```python
from build123d import *

# Parameters (mm, degrees)
SKETCH_1_W                  = 143.42529591
SKETCH_1_H                  = 80.35
SKETCH_1_R                  = 1.5
SKETCH_1_W_2                = 127.420983087
SKETCH_1_H_2                = 74.55
EXTRUDE_1_DEPTH             = 3
SKETCH_2_W                  = 131.42529591
SKETCH_2_H                  = 5
SKETCH_2_R                  = 1.5
EXTRUDE_2_DEPTH             = 2.8
SKETCH_3_R                  = 1.5
CUT_EXTRUDE_1_DEPTH         = 10
SKETCH_4_W                  = 6
SKETCH_4_H                  = 8
EXTRUDE_3_DEPTH             = 10
SKETCH_5_W                  = 54.485918212
SKETCH_5_H                  = 8
EXTRUDE_4_DEPTH             = 3
FILLET_1_R                  = 10
FILLET_2_R                  = 10
SKETCH_6_R                  = 1.5
CUT_EXTRUDE_2_DEPTH         = 3
EXTRUDE_5_DEPTH             = 2.8
SKETCH_8_W                  = 42.5
SKETCH_8_H                  = 8
SKETCH_8_H_2                = 10.9
SKETCH_8_R                  = 1.5
CUT_EXTRUDE_3_DEPTH         = 3
EXTRUDE_6_REACH             = 127.55
EXTRUDE_6_DIRECTION_2_DEPTH = 2.8
SKETCH_11_R                 = 1.5
SKETCH_11_R_2               = 1.490339558
CUT_EXTRUDE_4_DEPTH         = 3
EXTRUDE_START               = -3
EXTRUDE_7_DEPTH             = 3


with BuildPart() as part:
    # 草图1 → 凸台-拉伸1 (new body)
    with BuildSketch(Plane.XY):
        with Locations((-13.602517363, 6.11984421)):
            Rectangle(SKETCH_1_W, SKETCH_1_H)
        with Locations((55.610130592, -24.05515579)):
            Circle(SKETCH_1_R, mode=Mode.SUBTRACT)
        with Locations((55.610130592, 6.11984421)):
            Circle(SKETCH_1_R, mode=Mode.SUBTRACT)
        with Locations((55.610130592, 36.29484421)):
            Circle(SKETCH_1_R, mode=Mode.SUBTRACT)
        with Locations((-82.810852495, -24.05515579)):
            Circle(SKETCH_1_R, mode=Mode.SUBTRACT)
        with Locations((-82.810852495, 6.11984421)):
            Circle(SKETCH_1_R, mode=Mode.SUBTRACT)
        with Locations((-82.810852495, 36.29484421)):
            Circle(SKETCH_1_R, mode=Mode.SUBTRACT)
        with Locations((-13.600360952, 6.21984421)):
            Rectangle(SKETCH_1_W_2, SKETCH_1_H_2, mode=Mode.SUBTRACT)
    extrude(amount=EXTRUDE_1_DEPTH)

    # 草图2 → 凸台-拉伸2 (add)
    with BuildSketch(Plane(origin=(0, 46.29484421, 0), x_dir=(1, 0, 0), z_dir=(0, 1, 0))):
        with Locations((-13.602517363, -5.5)):
            Rectangle(SKETCH_2_W, SKETCH_2_H)
        with Locations(Location((-21.702517363, -5, 0), (0, 0, 180))):
            Circle(SKETCH_2_R, mode=Mode.SUBTRACT)
    extrude(amount=-EXTRUDE_2_DEPTH)

    # 草图3 → 切除-拉伸1 (cut)
    with BuildSketch(Plane(origin=(0, 46.29484421, 0), x_dir=(1, 0, 0), z_dir=(0, 1, 0))):
        with Locations(Location((0.240439338, -5, 0), (0, 0, 270))):
            Circle(SKETCH_3_R)
        with Locations(Location((-43.645478874, -5, 0), (0, 0, 270))):
            Circle(SKETCH_3_R)
    extrude(amount=-CUT_EXTRUDE_1_DEPTH, mode=Mode.SUBTRACT)

    # 草图4 → 凸台-拉伸3 (add)
    with BuildSketch(Plane(origin=(0, 46.29484421, 0), x_dir=(1, 0, 0), z_dir=(0, 1, 0))):
        with Locations((8.540439338, -4)):
            Rectangle(SKETCH_4_W, SKETCH_4_H)
        with Locations((-51.945478874, -4)):
            Rectangle(SKETCH_4_W, SKETCH_4_H)
    extrude(amount=EXTRUDE_3_DEPTH)

    # 草图5 → 凸台-拉伸4 (add)
    with BuildSketch(Plane(origin=(0, 56.29484421, 0), x_dir=(1, 0, 0), z_dir=(0, 1, 0))):
        with Locations((-21.702519768, -4)):
            Rectangle(SKETCH_5_W, SKETCH_5_H)
    extrude(amount=-EXTRUDE_4_DEPTH)

    # 圆角1
    fillet_1_edges = [part.edges().sort_by_distance(p)[0] for p in [
        (11.540439338, 46.29484421, 4),
        (-54.945478874, 46.29484421, 4),
    ]]
    fillet(fillet_1_edges, radius=FILLET_1_R - 0.0001)  # a hair under: the kernel refuses the full size

    # 圆角2
    fillet_2_edges = [part.edges().sort_by_distance(p)[0] for p in [
        (-54.945478874, 56.29484421, 4),
        (11.540439338, 56.29484421, 4),
    ]]
    fillet(fillet_2_edges, radius=FILLET_2_R)

    # 草图6 → 切除-拉伸2 (cut)
    with BuildSketch(Plane(origin=(0, 56.29484421, 0), x_dir=(1, 0, 0), z_dir=(0, 1, 0))):
        with Locations(Location((0.240439338, -5, 0), (0, 0, 270))):
            Circle(SKETCH_6_R)
        with Locations(Location((-21.702517363, -5, 0), (0, 0, 180))):
            Circle(SKETCH_6_R)
        with Locations(Location((-43.645478874, -5, 0), (0, 0, 270))):
            Circle(SKETCH_6_R)
    extrude(amount=-CUT_EXTRUDE_2_DEPTH, mode=Mode.SUBTRACT)

    # 草图7 → 凸台-拉伸5 (add)
    with BuildSketch(Plane(origin=(0, 46.29484421, 0), x_dir=(1, 0, 0), z_dir=(0, 1, 0))):
        with BuildLine():
            Line((52.110130592, -3), (-79.315165318, -3))
            ThreePointArc((-79.315165318, -3), (-71.408587337, -30.249323597), (-49.947485102, -48.808976146))
            ThreePointArc((-49.947485102, -48.808976146), (-47.931875984, -49.474706171), (-45.821160639, -49.7))
            Line((-45.821160639, -49.7), (3.801028521, -49.7))
            ThreePointArc((3.801028521, -49.7), (4.482979053, -49.676720076), (5.161754433, -49.606988694))
            ThreePointArc((5.161754433, -49.606988694), (36.42646247, -34.151078405), (52.110130592, -3))
        make_face()
    extrude(amount=-EXTRUDE_5_DEPTH)

    # 草图8 → 切除-拉伸3 (cut)
    with BuildSketch(Plane(origin=(0, 46.29484421, 0), x_dir=(1, 0, 0), z_dir=(0, 1, 0))):
        with BuildLine():
            Line((52.110130592, -8), (52.110130592, -3))
            ThreePointArc((52.110130592, -3), (51.686965751, -5.511139637), (51.148017839, -8))
            Line((51.148017839, -8), (52.110130592, -8))
        make_face()
        with BuildLine():
            ThreePointArc((-79.091069545, -8), (-79.253197971, -5.766605102), (-79.315165318, -3.528190833))
            Line((-79.315165318, -3.528190833), (-79.315165318, -8))
            Line((-79.315165318, -8), (-79.091069545, -8))
        make_face()
        with BuildLine():
            Line((-79.315165318, -3.528190833), (-79.315165318, -3))
            ThreePointArc((-79.315165318, -3), (-79.315862787, -3.264095416), (-79.315165318, -3.528190833))
        make_face()
        with Locations((-21.687503936, -23.091321672)):
            Rectangle(SKETCH_8_W, SKETCH_8_H)
        with Locations((-21.687503936, -13.641321672)):
            Rectangle(SKETCH_8_W, SKETCH_8_H_2)
        with Locations(Location((0.240439338, -5, 0), (0, 0, 270))):
            Circle(SKETCH_8_R)
        with Locations(Location((-43.645478874, -5, 0), (0, 0, 270))):
            Circle(SKETCH_8_R)
        with Locations(Location((-21.702517363, -5, 0), (0, 0, 270))):
            Circle(SKETCH_8_R)
    extrude(amount=-CUT_EXTRUDE_3_DEPTH, mode=Mode.SUBTRACT)

    # 凸台-拉伸6: up to this face of the body (flat: up to its plane)
    extrude_6_end = Plane(part.part.faces().sort_by_distance((-13.602517363, -34.05515579, 1.5))[0])
    # 草图9 → 凸台-拉伸6 (add, up to the picked face)
    with BuildSketch(Plane.XZ.offset(-43.49484421), mode=Mode.PRIVATE) as extrude_6_sk1:
        with BuildLine():
            ThreePointArc((-45.821160639, 49.7), (-47.931875984, 49.474706171), (-49.947485102, 48.808976146))
            ThreePointArc((-49.947485102, 48.808976146), (-71.265466668, 30.471277082), (-79.315165318, 3.528190833))
            Line((-79.315165318, 3.528190833), (-79.315165318, 3))
            Line((-79.315165318, 3), (-77.284463301, 3))
            Line((-77.284463301, 3), (-77.284463301, 5))
            ThreePointArc((-77.284463301, 5), (-69.179280492, 30.001857642), (-49.122220209, 46.987180917))
            ThreePointArc((-49.122220209, 46.987180917), (-47.509732915, 47.519764937), (-45.821160639, 47.7))
            Line((-45.821160639, 47.7), (3.801028521, 47.7))
            ThreePointArc((3.801028521, 47.7), (4.346588947, 47.681376061), (4.889609251, 47.625590956))
            ThreePointArc((4.889609251, 47.625590956), (34.185844829, 33.539377025), (49.748453895, 5))
            Line((49.748453895, 5), (50.110130592, 3))
            Line((50.110130592, 3), (52.615296987, 3))
            ThreePointArc((52.615296987, 3), (38.28835989, 32.947499211), (9.430945753, 49.359795972))
            ThreePointArc((9.430945753, 49.359795972), (7.851760578, 49.614706494), (6.254409581, 49.7))
            Line((6.254409581, 49.7), (-45.821160639, 49.7))
        make_face()
    extrude_6_tool1 = split(extrude(extrude_6_sk1.sketch, amount=EXTRUDE_6_REACH, mode=Mode.PRIVATE), bisect_by=extrude_6_end, keep=Keep.BOTH, mode=Mode.PRIVATE)
    add(extrude_6_tool1.solids().sort_by(Axis((-47.636477, 43.494844, 48.106717), (0, -1, 0)))[0])

    # 草图9 → 凸台-拉伸6 direction 2 (add)
    with BuildSketch(Plane.XZ.offset(-43.49484421)):
        with BuildLine():
            ThreePointArc((-45.821160639, 49.7), (-47.931875984, 49.474706171), (-49.947485102, 48.808976146))
            ThreePointArc((-49.947485102, 48.808976146), (-71.265466668, 30.471277082), (-79.315165318, 3.528190833))
            Line((-79.315165318, 3.528190833), (-79.315165318, 3))
            Line((-79.315165318, 3), (-77.284463301, 3))
            Line((-77.284463301, 3), (-77.284463301, 5))
            ThreePointArc((-77.284463301, 5), (-69.179280492, 30.001857642), (-49.122220209, 46.987180917))
            ThreePointArc((-49.122220209, 46.987180917), (-47.509732915, 47.519764937), (-45.821160639, 47.7))
            Line((-45.821160639, 47.7), (3.801028521, 47.7))
            ThreePointArc((3.801028521, 47.7), (4.346588947, 47.681376061), (4.889609251, 47.625590956))
            ThreePointArc((4.889609251, 47.625590956), (34.185844829, 33.539377025), (49.748453895, 5))
            Line((49.748453895, 5), (50.110130592, 3))
            Line((50.110130592, 3), (52.615296987, 3))
            ThreePointArc((52.615296987, 3), (38.28835989, 32.947499211), (9.430945753, 49.359795972))
            ThreePointArc((9.430945753, 49.359795972), (7.851760578, 49.614706494), (6.254409581, 49.7))
            Line((6.254409581, 49.7), (-45.821160639, 49.7))
        make_face()
    extrude(amount=-EXTRUDE_6_DIRECTION_2_DEPTH)

    # 草图11 → 切除-拉伸4 (cut)
    with BuildSketch(Plane(origin=(0, 0, 47.7), x_dir=(-1, 0, 0), z_dir=(0, 0, -1))):
        with Locations((15.702514958, 40.59484421)):
            Circle(SKETCH_11_R)
        with Locations((27.702514958, 40.59484421)):
            Circle(SKETCH_11_R)
        with Locations((15.702514958, 28.59484421)):
            Circle(SKETCH_11_R)
        with Locations((27.702514958, 28.59484421)):
            Circle(SKETCH_11_R_2)
        with Locations((27.702514958, 16.59484421)):
            Circle(SKETCH_11_R)
        with Locations((15.702514958, 16.59484421)):
            Circle(SKETCH_11_R)
    extrude(amount=-CUT_EXTRUDE_4_DEPTH, mode=Mode.SUBTRACT)

    # 草图12 → 凸台-拉伸7 (add)
    with BuildSketch(Plane.XZ.offset(34.05515579).offset(EXTRUDE_START)):
        with BuildLine():
            Line((50.110130592, 3), (-77.284463301, 3))
            Line((-77.284463301, 3), (-77.284463301, 5))
            ThreePointArc((-77.284463301, 5), (-69.179280492, 30.001857642), (-49.122220209, 46.987180917))
            ThreePointArc((-49.122220209, 46.987180917), (-47.509732915, 47.519764937), (-45.821160639, 47.7))
            Line((-45.821160639, 47.7), (3.801028521, 47.7))
            ThreePointArc((3.801028521, 47.7), (4.346588947, 47.681376061), (4.889609251, 47.625590956))
            ThreePointArc((4.889609251, 47.625590956), (34.185844829, 33.539377025), (49.748453895, 5))
            Line((49.748453895, 5), (50.110130592, 3))
        make_face()
        with BuildLine():
            Line((50.110130592, 3), (52.110130592, 3))
            Line((52.110130592, 3), (52.615296987, 3))
            ThreePointArc((52.615296987, 3), (38.28835989, 32.947499211), (9.430945753, 49.359795972))
            ThreePointArc((9.430945753, 49.359795972), (7.851760578, 49.614706494), (6.254409581, 49.7))
            Line((6.254409581, 49.7), (3.801028521, 49.7))
            Line((3.801028521, 49.7), (-45.821160639, 49.7))
            ThreePointArc((-45.821160639, 49.7), (-47.931875984, 49.474706171), (-49.947485102, 48.808976146))
            ThreePointArc((-49.947485102, 48.808976146), (-71.265466668, 30.471277082), (-79.315165318, 3.528190833))
            Line((-79.315165318, 3.528190833), (-79.315165318, 3))
            Line((-79.315165318, 3), (-77.284463301, 3))
            Line((-77.284463301, 3), (-77.284463301, 5))
            ThreePointArc((-77.284463301, 5), (-69.179280492, 30.001857642), (-49.122220209, 46.987180917))
            ThreePointArc((-49.122220209, 46.987180917), (-47.509732915, 47.519764937), (-45.821160639, 47.7))
            Line((-45.821160639, 47.7), (3.801028521, 47.7))
            ThreePointArc((3.801028521, 47.7), (4.346588947, 47.681376061), (4.889609251, 47.625590956))
            ThreePointArc((4.889609251, 47.625590956), (34.185844829, 33.539377025), (49.748453895, 5))
            Line((49.748453895, 5), (50.110130592, 3))
        make_face()
    extrude(amount=EXTRUDE_7_DEPTH)


solid = part.part
```
Verification items for the finished model (mm, model axes). A direction names the side the tool comes from. Coordinates: 2 decimals unless noted, no trailing zeros. Loops run counter-clockwise (first coordinate to the right, second up) from the corner with the lowest first, then second, coordinate; pieces in that order, holes last. Notation, with made-up numbers: (11, 54.5) -> (40, 54.5) arc R24 ccw to (40, 90.5) -> close; hole circle Ø10 at (12.25, 29). An arc over 180 degrees is marked (long way). Answer in a Markdown table with one row per item.
1) Section check A-A (x = -34.5). Record the cut outline in (y, z).
The answers:
| item | result |
|---|---|
| outline | (-34.06, 0) -> (-31.06, 0) -> (-31.06, 47.7) -> (43.49, 47.7) -> (43.49, 27.09) -> (46.29, 27.09) -> (46.29, 49.7) -> (-34.06, 49.7) -> close; (43.49, 0) -> (46.29, 0) -> (46.29, 8.19) -> (43.49, 8.19) -> close; (53.29, 0) -> (56.29, 0) -> (56.29, 8) -> (53.29, 8) -> close |
2) Draft check along Z on faces 5 (the face through (-22, 45, 27.091)), 6 (the face through (-15, 46.295, 30)), 7 (the face through (-19, 7, 49.7)). Enter one of: released by +Z, released by -Z, zero draft, split by the parting line, or undercut.
The answers:
| item | result |
|---|---|
| face 5 | undercut |
| face 6 | zero draft |
| face 7 | released by +Z |
3) Depth check by flat-ended pin: P1, Ø3, axis at y = 45.5, z = 16.5, coming from the -X side; P2, Ø12, axis at x = -67, z = 6.5, coming from the +Y side; P3, Ø14.5, axis at x = 13, z = 31, coming from the +Y side; P4, Ø5, axis at x = 55.61, y = 36.29, coming from the -Z side. Enter the tip coordinate at first touch or a pass-through.
The answers:
| item | result |
|---|---|
| P1 | stops at x = -77.92 |
| P2 | stops at y = 47.11 |
| P3 | stops at y = 46.29 |
| P4 | stops at z = 0 |
4) Access from +Z, -Z, +X, -X, +Y, -Y to the whole of each face (thin tool, end or side, straight path). Record for faces 1 (the face through (-22, 45, 8.191)), 2 (the face through (5.54, 50, 4)), 3 (the face through (-21, 7, 47.7)), 4 (the face through (-22, 54, 8)).
The answers:
| item | result |
|---|---|
| face 1 | +Y |
| face 2 | +Z, -Z |
| face 3 | -Z |
| face 4 | +Z, +X, -X, +Y |
5) Section check B-B (z = 32). Record the cut outline in (x, y).
The answers:
| item | result |
|---|---|
| outline | (-70.23, -34.06) -> (39.15, -34.06) -> (39.15, 46.29) -> (-70.23, 46.29) -> close; hole (-67.76, -31.06) -> (35.74, -31.06) -> (35.74, 43.49) -> (-67.76, 43.49) -> close |
6) Scan lines: line 1 along Y through (x, z) = (-42, 6); line 2 along Y through (x, z) = (-11, 35.5); line 3 along X through (y, z) = (45.25, 5). Record each from-to range of solid material in increasing order. Write a range as from..to.
The answers:
| item | result |
|---|---|
| line 1 | y = -34.06..-31.06, 43.49..46.29, 53.29..56.29 |
| line 2 | y = -34.06..-31.06, 43.49..46.29 |
| line 3 | x = -79.29..-45.15, -42.15..-23.2, -20.2..-1.26, 1.74..52.29 |
7) Section check C-C (x = 41). Record the cut outline in (y, z).
The answers:
| item | result |
|---|---|
| outline | (-34.06, 0) -> (-31.06, 0) -> (-31.06, 25.65) -> (43.49, 25.65) -> (43.49, 0) -> (46.29, 0) -> (46.29, 29.81) -> (-34.06, 29.81) -> close |
